Part model, mm, in its own coordinate system. Face numbers are marked on the shaded views. A direction names the side the tool comes from. Give positions to 0.01 mm unless a question says otherwise; leave off trailing zeros. Order: outer loops, then holes, each group sorted by start corner. A loop starts at its lowest first (then second) coordinate and runs counter-clockwise, first axis right, second up. Notation, with made-up numbers: M 49.25,86.5 L 90.25,86.5 A24 ccw 90.25,115.5 Z; hole C 49.5,30.5 d4. An arc over 180 degrees is marked long. One line per question, with ' | ' between items.
```python
from build123d import *

# Parameters (mm, degrees)
F0_R           = 17.78
F1_DEPTH       = 10.16
F3_D           = 5.1054
F3_CSINK_D     = 10.4394
F3_CSINK_ANGLE = 82
F5_DEPTH       = 11.43
F4_R           = 6.35
F6_DEPTH       = 4.445
F7_SIZE        = 5.08


with BuildPart() as f1:
    # F0 (on Top) → F1 (new body)
    with BuildSketch(Plane.XY):
        Circle(F0_R)
    extrude(amount=F1_DEPTH)

    # F3 (through all)
    with Locations(Plane.XY.offset(10.16)):
        with Locations((0, 0)):
            CounterSinkHole(F3_D / 2, F3_CSINK_D / 2, counter_sink_angle=F3_CSINK_ANGLE)

    # F4 (on Top) → F5 (join)
    with BuildSketch(Plane.XY):
        with BuildLine():
            Line((5.0501466563, 7.3162913248), (7.9375, 7.3162913248))
            ThreePointArc((7.9375, 7.3162913248), (0, 10.795), (-7.9375, 7.3162913248))
            Line((-7.9375, 7.3162913248), (-5.0501466563, 7.3162913248))
            ThreePointArc((-5.0501466563, 7.3162913248), (0, 8.89), (5.0501466563, 7.3162913248))
        make_face()
        with BuildLine():
            Line((7.9375, 4.0035226676), (7.9375, 7.3162913248))
            Line((7.9375, 7.3162913248), (5.0501466563, 7.3162913248))
            ThreePointArc((5.0501466563, 7.3162913248), (6.7017423452, 5.8411257082), (7.9375, 4.0035226676))
        make_face()
        with BuildLine():
            Line((-5.0501466563, 7.3162913248), (-7.9375, 7.3162913248))
            Line((-7.9375, 7.3162913248), (-7.9375, 4.0035226676))
            ThreePointArc((-7.9375, 4.0035226676), (-6.7017423452, 5.8411257082), (-5.0501466563, 7.3162913248))
        make_face()
        with BuildLine():
            Line((-7.9375, -4.0035226676), (-7.9375, -7.3162913248))
            Line((-7.9375, -7.3162913248), (-5.0501466563, -7.3162913248))
            ThreePointArc((-5.0501466563, -7.3162913248), (-6.7017423452, -5.8411257082), (-7.9375, -4.0035226676))
        make_face()
        with BuildLine():
            ThreePointArc((-7.9375, -7.3162913248), (0, -10.795), (7.9375, -7.3162913248))
            Line((7.9375, -7.3162913248), (5.0501466563, -7.3162913248))
            ThreePointArc((5.0501466563, -7.3162913248), (0, -8.89), (-5.0501466563, -7.3162913248))
            Line((-5.0501466563, -7.3162913248), (-7.9375, -7.3162913248))
        make_face()
        with BuildLine():
            Line((5.0501466563, -7.3162913248), (7.9375, -7.3162913248))
            Line((7.9375, -7.3162913248), (7.9375, -4.0035226676))
            ThreePointArc((7.9375, -4.0035226676), (6.7017423452, -5.8411257082), (5.0501466563, -7.3162913248))
        make_face()
    extrude(amount=-F5_DEPTH)

    # F4 (on Top) → F6 (join)
    with BuildSketch(Plane.XY):
        with BuildLine():
            ThreePointArc((7.9375, 4.0035226676), (6.7017423452, 5.8411257082), (5.0501466563, 7.3162913248))
            Line((5.0501466563, 7.3162913248), (-5.0501466563, 7.3162913248))
            ThreePointArc((-5.0501466563, 7.3162913248), (-6.7017423452, 5.8411257082), (-7.9375, 4.0035226676))
            Line((-7.9375, 4.0035226676), (-7.9375, -4.0035226676))
            ThreePointArc((-7.9375, -4.0035226676), (-6.7017423452, -5.8411257082), (-5.0501466563, -7.3162913248))
            Line((-5.0501466563, -7.3162913248), (5.0501466563, -7.3162913248))
            ThreePointArc((5.0501466563, -7.3162913248), (6.7017423452, -5.8411257082), (7.9375, -4.0035226676))
            Line((7.9375, -4.0035226676), (7.9375, 4.0035226676))
        make_face()
        Circle(F4_R, mode=Mode.SUBTRACT)
        with BuildLine():
            ThreePointArc((-5.0501466563, -7.3162913248), (0, -8.89), (5.0501466563, -7.3162913248))
            Line((5.0501466563, -7.3162913248), (-5.0501466563, -7.3162913248))
        make_face()
        with BuildLine():
            Line((-5.0501466563, 7.3162913248), (5.0501466563, 7.3162913248))
            ThreePointArc((5.0501466563, 7.3162913248), (0, 8.89), (-5.0501466563, 7.3162913248))
        make_face()
    extrude(amount=-F6_DEPTH)

    # F7
    f7_edges = [f1.edges().sort_by_distance(p)[0] for p in [
        (-17.78, 0, 10.16),
    ]]
    chamfer(f7_edges, length=F7_SIZE)


solid = f1.part
```
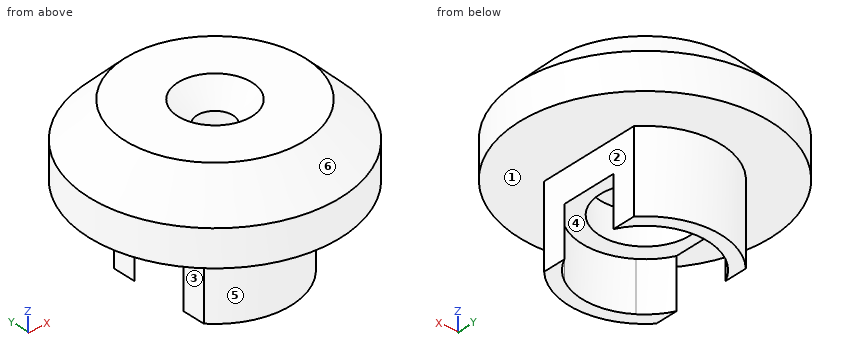
1. Drop flat-ended pins along their axis: pin 1 (2 mm diameter, centred on y = -1, z = -4.5, fed in from -X); pin 2 (12.5 mm diameter, centred on x = -1, y = -0.5, fed in from -Z) (3 decimals); pin 3 (6.5 mm diameter, centred on x = 2, y = 1.5, fed in from -Z). Give the stop position or say it passes through.
Worked out:
pin 1: stops at x = -7.94 | pin 2: stops at z = -4.445 | pin 3: stops at z = 0
2. Slice it at D-D on z = 6.5. Give the cut face in (x, y).
Worked out:
outline: C 0,0 d32.72; hole C 0,0 d5.11
3. Mould opens along Y. For the marked faces 4, 5 and 6 say: released by +Y, released by -Y, zero draft, split by the parting line, or undercut.
Worked out:
face 4: undercut | face 5: released by -Y | face 6: split by the parting line
4. Tool access for the marked faces 1, 2 and 3: list every direction of +Z, -Z, +X, -X, +Y, -Y with a clear straight run to the whole face (end or side of a thin tool).
Worked out:
face 1: -Z | face 2: -Z, +X, +Y, -Y | face 3: -Z, -X, +Y, -Y
5. Slice it at A-A on x = 0. Give the cut face in (y, z) (3 decimals), then the cut area to 3 significant figures.
Worked out:
outline: M -17.78,0 L -10.795,0 L -10.795,-11.43 L -8.89,-11.43 L -8.89,-4.445 L -6.35,-4.445 L -6.35,0 L -2.553,0 L -2.553,7.092 L -5.22,10.16 L -12.7,10.16 L -17.78,5.08 Z; M 2.553,0 L 6.35,0 L 6.35,-4.445 L 8.89,-4.445 L 8.89,-11.43 L 10.795,-11.43 L 10.795,0 L 17.78,0 L 17.78,5.08 L 12.7,10.16 L 5.22,10.16 L 2.553,7.092 Z | area: 342 mm2
6. Probe L1, parallel to Y at x = 0, z = 3.75; L2, parallel to Z at x = -6, y = -5.5 (3 decimals); L3, parallel to X at y = 2, z = 7.5. List the from-to ranges inside material, lowest first. Write a range as from..to.
Worked out:
L1: y = -17.78..-2.55, 2.55..17.78 | L2: z = -4.445..10.16 | L3: x = -15.23..-2.11, 2.11..15.23
